Design review of the part built by this model. Coordinates are the model's own, in mm. A direction names the side the tool comes from. Give positions to 0.01 mm unless a question says otherwise; leave off trailing zeros. Order: outer loops, then holes, each group sorted by start corner. A loop starts at its lowest first (then second) coordinate and runs counter-clockwise, first axis right, second up. Notation, with made-up numbers: (56.5, 65) -> (82.5, 65) arc R22 ccw to (82.5, 74) -> close; hole circle Ø7 at (82.5, 12.5). An arc over 180 degrees is marked (long way). One line per item, written item: value.
Autodesk Inventor part; units mm, degrees
ref_plane "YZ Plane" through (0, 0, 0) normal (1, 0, 0) x (0, 1, 0)
ref_plane "XZ Plane" through (0, 0, 0) normal (0, 1, 0) x (-1, 0, 0)
ref_plane "XY Plane" through (0, 0, 0) normal (0, 0, 1) x (1, 0, 0)
sketch "Эскиз1" plane through (0, 0, 0) normal (1, 0, 0) x (0, 1, 0)
  line L0 (-270, 200) -> (330, 200)
  line L1 (330, 200) -> (330, -200)
  line L2 (330, -200) -> (-270, -200)
  line L3 (-270, -200) -> (-270, 200)
  line L4 (-270, 200) -> (330, -200) construction
  line L5 (330, 200) -> (-270, -200) construction
  point P0 (30, 0)
  point P1 (0, 0)
  dimension "d0" = 400
  dimension "d1" = 600
  dimension "d73" = 30
extrude "Выдавливание1" add sketch "Эскиз1" along normal blind 50
sketch "Эскиз3" plane through (50, 0, 0) normal (1, 0, 0) x (0, 0, -1)
  line L0 (-200, 330) -> (-200, -270)
  line L1 (-200, -270) -> (200, -270)
  line L2 (-200, 330) -> (-196, 330)
  line L3 (-196, 330) -> (-196, -270)
  line L4 (-196, -270) -> (-200, -270)
  line L5 (-200, -270) -> (-200, 330)
  line L6 (200, 330) -> (-200, 330)
  line L7 (200, -270) -> (196, -270)
  line L8 (196, -270) -> (196, 330)
  line L9 (196, 330) -> (200, 330)
  line L10 (200, 330) -> (200, -270)
  line L11 (200, -270) -> (200, 330)
  line L12 (-200, 330) -> (200, 330)
  line L13 (200, 330) -> (200, 326)
  line L14 (200, 326) -> (-200, 326)
  line L15 (-200, 326) -> (-200, 330)
  point P0 (0, 0)
  point P1 (-196, 326)
  point P2 (196, 326)
  dimension "d74" = 4
  dimension "d75" = 4
  dimension "d76" = 4
extrude "Выдавливание3" cut sketch "Эскиз3" against normal blind 20 contours L2 L3 L14 L0 | L14 L3 L1 L0 | L6 L8 L14 L3 | L6 L10 L14 L8 | L14 L10 L1 L8
sketch "Эскиз4" plane through (50, 0, 0) normal (1, 0, 0) x (0, 0, -1)
  line L0 (68.9117, -237) -> (68.9117, -247) construction
  line L1 (38.9117, -237) -> (38.9117, -247) construction
  line L2 (58.9117, -237) -> (58.9117, -247) construction
  line L3 (58.9117, -237) -> (68.9117, -237) construction
  line L4 (68.9117, -247) -> (58.9117, -247) construction
  line L5 (68.9117, -247) -> (88.9117, -247) construction
  line L6 (88.9117, -237) -> (68.9117, -237) construction
  line L7 (88.9117, -247) -> (88.9117, -237) construction
  line L8 (98.9117, -237) -> (98.9117, -247) construction
  line L9 (88.9117, -237) -> (98.9117, -237) construction
  line L10 (98.9117, -247) -> (88.9117, -247) construction
  line L11 (38.9117, -247) -> (28.9117, -247) construction
  line L12 (28.9117, -237) -> (38.9117, -237) construction
  line L13 (28.9117, -247) -> (28.9117, -237) construction
  line L14 (28.9117, -237) -> (8.9117, -237) construction
  line L15 (28.9117, -247) -> (28.9117, -237) construction
  line L16 (28.9117, -237) -> (8.9117, -237) construction
  line L17 (8.9117, -237) -> (8.9117, -247) construction
  line L18 (8.9117, -247) -> (28.9117, -247) construction
  line L19 (-1.0883, -237) -> (8.9117, -237) construction
  line L20 (-1.0883, -237) -> (-1.0883, -247) construction
  line L21 (8.9117, -247) -> (-1.0883, -247) construction
  line L22 (8.9117, -237) -> (8.9117, -247) construction
  line L23 (53.9117, -250) -> (43.9117, -250)
  line L24 (43.9117, -250) -> (43.9117, 276)
  line L25 (43.9117, 276) -> (53.9117, 276)
  line L26 (53.9117, 276) -> (53.9117, -250)
  line L27 (196, 326) -> (-196, 326)
  line L28 (-196, -270) -> (196, -270)
  point P0 (0, 0)
  dimension "d80" = 15
  dimension "d81" = 15
  dimension "d82" = 50
  dimension "d83" = 20
extrude "Выдавливание4" cut sketch "Эскиз4" against normal blind 60
sketch "Эскиз5" plane through (50, 0, 0) normal (1, 0, 0) x (0, 0, -1)
  line L0 (-89.8865, 149.6936) -> (-99.7391, 147.983)
  line L1 (-99.7391, 147.983) -> (-100.4234, 151.9241)
  line L2 (-100.4234, 151.9241) -> (-90.5708, 153.6347)
  line L3 (-90.5708, 153.6347) -> (-89.8865, 149.6936)
  line L4 (-132.1786, 222.6367) -> (-133.7515, 226.3145)
  line L5 (-133.7515, 226.3145) -> (-124.5571, 230.2467)
  line L6 (-124.5571, 230.2467) -> (-122.9842, 226.5689)
  line L7 (-122.9842, 226.5689) -> (-132.1786, 222.6367)
  line L8 (-109.4825, 186.8162) -> (-109.4497, 190.8161)
  line L9 (-109.4497, 190.8161) -> (-99.45, 190.734)
  line L10 (-99.45, 190.734) -> (-99.4828, 186.7341)
  line L11 (-99.4828, 186.7341) -> (-109.4825, 186.8162)
  line L12 (-101.3444, 227.5816) -> (-102.6741, 223.8091)
  line L13 (-102.6741, 223.8091) -> (-112.1054, 227.1332)
  line L14 (-112.1054, 227.1332) -> (-110.7758, 230.9058)
  line L15 (-110.7758, 230.9058) -> (-101.3444, 227.5816)
  line L16 (-121.5737, 151.067) -> (-130.5132, 155.5487)
  line L17 (-130.5132, 155.5487) -> (-128.7205, 159.1245)
  line L18 (-128.7205, 159.1245) -> (-119.781, 154.6428)
  line L19 (-119.781, 154.6428) -> (-121.5737, 151.067)
  line L20 (-73.3529, 162.3525) -> (-66.0686, 169.2037)
  line L21 (-66.0686, 169.2037) -> (-63.3281, 166.29)
  line L22 (-63.3281, 166.29) -> (-70.6124, 159.4388)
  line L23 (-70.6124, 159.4388) -> (-73.3529, 162.3525)
  line L24 (-146.4475, 202.9259) -> (-150.1162, 204.5198)
  line L25 (-150.1162, 204.5198) -> (-146.1314, 213.6916)
  line L26 (-146.1314, 213.6916) -> (-142.4627, 212.0976)
  line L27 (-142.4627, 212.0976) -> (-146.4475, 202.9259)
  line L28 (-88.6954, 198.226) -> (-94.2983, 189.943)
  line L29 (-94.2983, 189.943) -> (-97.6115, 192.1842)
  line L30 (-97.6115, 192.1842) -> (-92.0086, 200.4671)
  line L31 (-92.0086, 200.4671) -> (-88.6954, 198.226)
  line L32 (-87.8306, 208.7569) -> (-91.5842, 207.3746)
  line L33 (-91.5842, 207.3746) -> (-95.04, 216.7585)
  line L34 (-95.04, 216.7585) -> (-91.2865, 218.1408)
  line L35 (-91.2865, 218.1408) -> (-87.8306, 208.7569)
  line L36 (-142.6786, 173.9561) -> (-146.3858, 172.4539)
  line L37 (-146.3858, 172.4539) -> (-150.1413, 181.7219)
  line L38 (-150.1413, 181.7219) -> (-146.434, 183.2241)
  line L39 (-146.434, 183.2241) -> (-142.6786, 173.9561)
  line L40 (-57.2, 186.602) -> (-55.7515, 196.4965)
  line L41 (-55.7515, 196.4965) -> (-51.7937, 195.9171)
  line L42 (-51.7937, 195.9171) -> (-53.2422, 186.0226)
  line L43 (-53.2422, 186.0226) -> (-57.2, 186.602)
  circle A0 centre (-110, 199.3849) radius 60
  point P0 (0, 0)
hole "Отверстие1" at (50, 199.3849, 110) direction (-1, 0, 0) diameter 8.1 depth 80
sketch "Эскиз6" plane through (50, 0, 0) normal (1, 0, 0) x (0, 0, -1)
  line L0 (-196, 326) -> (-196, -270)
  line L1 (-196, 326) -> (196, 326)
  line L2 (196, 326) -> (196, 320)
  line L3 (196, 320) -> (-196, 320)
  line L4 (-196, 320) -> (-196, 326)
  point P0 (0, 0)
  dimension "d93" = 6
  dimension "d94" = 392
extrude "Выдавливание5" add sketch "Эскиз6" along normal blind 70
properties part number "Общий концепт в 3д"
Item 1: Add section B-B on z = 61.5. Give the boundary of the cut face in (x, y).
Returned:
outline: (0, -270) -> (50, -270) -> (50, 320) -> (120, 320) -> (120, 326) -> (30, 326) -> (30, 330) -> (0, 330) -> close
Item 2: Add section A-A on y = 244. Give the boundary of the cut face in (x, z), plus the area to 3 significant figures.
Returned:
outline: (0, -200) -> (30, -200) -> (30, -196) -> (50, -196) -> (50, -53.91) -> (0, -53.91) -> close; (0, -43.91) -> (50, -43.91) -> (50, 196) -> (30, 196) -> (30, 200) -> (0, 200) -> close
area: 19,300 mm²
Item 3: Draft analysis for pull direction Z (two halves, no side actions). For faces 1 (the flat face through (25, -270, -3)), 2 (the flat face through (25, 17, -53.912)), 3 (the flat face through (15, 26, 200)), state which applies: pulls with the +Z half, pulls with the -Z half, needs draft (parallel to the pull), parting line crosses it, or undercut.
Returned:
face 1: needs draft
face 2: undercut
face 3: pulls with the +Z half
Item 4: Add section C-C on x = 106.5. Give the boundary of the cut face in (y, z), plus the area to 3 significant figures.
Returned:
outline: (320, -196) -> (326, -196) -> (326, 196) -> (320, 196) -> close
area: 2,350 mm²
Item 5: Machinability: for faces 4 (the flat face through (38, 29, -196)), 5 (the flat face through (74, 326, 3)), 6 (the flat face through (25, 9, -43.912)), 7 (the flat face through (38, 29, 196)), 8 (the flat face through (50, 21, 3)), which of the approach directions +Z, -Z, +X, -X, +Y, -Y give a long, thin tool a straight path to every point of the face, cutting with its end or side? Answer none if there is none.
Returned:
face 4: -Z, +X, +Y, -Y
face 5: +Z, -Z, +X, +Y
face 6: +X, -X
face 7: +Z, +X, +Y, -Y
face 8: +Z, -Z, +X, -Y
Item 6: Clearance check with flat-ended pins moving along their axes: P1, Ø3, axis at y = 158, z = -1.5, coming from the +X side; P2, Ø21, axis at x = 84, z = -77.5, coming from the -Y side; P3, Ø6.5, axis at y = 199.38, z = 110, coming from the -X side. State where each tip first meets the part, or that it passes through.
Returned:
P1: x = 50
P2: y = 320
P3: through
Item 7: To check wall thickness, follow line 1 along Z through (x, y) = (23, -92.5); line 2 along Z through (x, y) = (47.5, 91); line 3 along Y through (x, z) = (13, 110). State the ranges of each line that lie inside material, in increasing order. Write a range as from..to.
Returned:
line 1: -200..-53.91, -43.91..200
line 2: -196..-53.91, -43.91..196
line 3: -270..195.33, 203.43..330
